Solid Edge part; units mm, degrees
sketch "Sketch1" plane through (0, 0, 0) normal (0, 0, 1) x (1, 0, 0)
  circle A0 centre (0, 0) radius 6
extrude "Protrusion1" add sketch "Sketch1" along normal blind 3.3
sketch "Sketch2" plane through (0, 0, 0) normal (0, 0, -1) x (1, 0, 0)
  circle A0 centre (0, 0) radius 3
extrude "Protrusion2" add sketch "Sketch2" along normal blind 56.7
sketch "Sketch3" plane through (0, 0, -56.7) normal (0, 0, -1) x (1, 0, 0)
  circle A0 centre (0, 0) radius 2.9997
extrude "Cutout1" cut sketch "Sketch3" against normal blind 18 flip side to cut
chamfer "Chamfer_1" distance 0.45 angle 45 1 edges at (-2.9997, 0, -56.7)
sketch "Sketch4" plane through (0, 0, 3.3) normal (0, 0, 1) x (1, 0, 0)
  line L0 (-1.1547, 2) -> (1.1547, 2)
  line L1 (2.3094, 0) -> (1.1547, 2)
  line L2 (1.1547, -2) -> (2.3094, 0)
  line L3 (-1.1547, -2) -> (1.1547, -2)
  line L4 (-2.3094, 0) -> (-1.1547, -2)
  line L5 (-1.1547, 2) -> (-2.3094, 0)
extrude "Cutout2" cut sketch "Sketch4" against normal blind 2.2
sketch "Sketch5" plane through (0, 0, 0) normal (0, -1, 0) x (1, 0, 0)
  line L0 (6, 3.3) -> (2.7, 0)
  line L1 (2.7, 0) -> (6, 0)
  line L2 (6, 0) -> (6, 3.3)
revolve "RevolvedCutout1" cut sketch "Sketch5" angle 360 about axis through (0, 0, 14.0017) along (0, 0, -1)
properties part number "209564" material "Stainless Steel, 304"
Work out the finished part from the listing and answer in its coordinate system (mm). A direction names the side the tool comes from. Give positions to 0.01 mm unless a question says otherwise; leave off trailing zeros. Loops run counter-clockwise (first coordinate to the right, second up) from the corner with the lowest first, then second, coordinate; pieces in that order, holes last. Notation, with made-up numbers: M 80.25,36.25 L 110.25,36.25 A15 cw 110.25,44.25 Z; hole C 7,-5.5 d3. An arc over 180 degrees is marked long. Use CSV: the item, a comma, the result in double quotes.
1) Determine the mould class of faces 1 (the flat face through (0, 0, -56.7)), 2 (the flat face through (0, 0, 1.1)), 3 (the flat face through (0, -2, 2)), 4 (the cylindrical face through (-3, 0, -19)) for opening direction X: released by +X, released by -X, zero draft, split by the parting line, or undercut.
Answer:
face 1,"zero draft"
face 2,"undercut"
face 3,"undercut"
face 4,"split by the parting line"
2) Find section B-B on z = -19. Write down the section's boundary in (x, y), plus the area to 3 significant figures.
Answer:
outline,"C 0,0 d6"
area,"28.3 mm^2"
3) Which of the six approach directions +Z, -Z, +X, -X, +Y, -Y give full straight-line access (tool end or side, diameter ignored) to faces 5 (the flat face through (-1.74, -0.99, 2.22)), 6 (the cylindrical face through (2.86, -0.9, -47.6)), 7 (the flat face through (3, 0, 3.3))?
Answer:
face 5,"+Z"
face 6,"-Z"
face 7,"+Z, +X, -X, +Y, -Y"
4) Consider L1, parallel to Y at x = 0.25, z = -18; L2, parallel to X at y = 2.25, z = -53; L3, parallel to Z at x = 0.25, y = -1.75. Determine where each line is inside the solid, lowest interval first.
Answer:
L1,"-2.99 to 2.99"
L2,"-1.98 to 1.98"
L3,"-56.7 to 1.1"
5) Given P1, Ø5, axis at y = 3.5, z = -7, coming from the -X side; P2, Ø1.5, axis at x = -4.5, z = -4, coming from the -Y side (3 decimals); P3, Ø1.8, axis at x = 0, z = 2, coming from the -Y side; P4, Ø1, axis at x = -2.5, z = -27, coming from the +Y side, each flat-ended and moving along its own axis, determine where each tip first touches the part or whether it passes through.
Answer:
P1,"x = -2.83"
P2,"through"
P3,"y = -5.6"
P4,"y = 2.24"
